The listing builds one solid part. Answer for the finished solid, in the listing's coordinates (mm). Coordinates: 2 decimals unless noted, no trailing zeros. Return JSON: item names as keys, results as strings.
Autodesk Inventor part; units mm, degrees
ref_plane "Work Plane1" through (0, 1.5, 0) normal (0, 1, 0) x (1, 0, 0)
ref_plane "YZ Plane" through (0, 0, 0) normal (1, 0, 0) x (0, 1, 0)
ref_plane "XZ Plane" through (0, 0, 0) normal (0, 1, 0) x (-1, 0, 0)
sketch "Sketch1" plane through (0, 0, 0) normal (0, 1, 0) x (-1, 0, 0)
  circle A0 centre (0, 0) radius 7.5
  dimension "d0" = 15
extrude "Extrusion1" add sketch "Sketch1" along normal blind 1
ref_plane "Work Plane1" through (0, 1.5, 0) normal (0, 1, 0) x (1, 0, 0)
sketch "Sketch3" plane through (0, 1.5, 0) normal (0, 1, 0) x (1, 0, 0)
  circle A0 centre (0, 0) radius 1.6
  dimension "d7" = 3.2
extrude "Extrusion3" cut sketch "Sketch3" against normal up to surface (1.5 mm away)
fillet "Fillet2" radius 0.5 2 edges at (7.5, 0, 0) (7.5, 1, 0)
chamfer "Chamfer2" distance 0.25 angle 45 2 edges at (-1.6, 0, 0) (-1.6, 1, 0)
properties part number "BoxWasher"
1. Consider line 1 (Z direction, x = 0, y = 0.55); line 2 (X direction, y = 0.15, z = 5.75); line 3 (Z direction, x = -3, y = 0.65). Determine where each line is inside the solid, lowest interval first. Write a range as from..to.
Answer block:
{"line 1": "z = -7.5..-1.6, 1.6..7.5", "line 2": "x = -4.59..4.59", "line 3": "z = -6.85..6.85"}
2. This flat-tipped pin is pushed along its axis until it touches: pin 1 Ø3.5 at (x, z) = (0, 0) entering from +Y. Where does it stop, or does it pass through?
Answer block:
{"pin 1": "stops at y = 0.9"}
3. Determine the mould class of faces 1 (the face through (-1.27, 0.5, 0.97)), 2 (the face through (-1.5, 1, -1.5)) for opening direction Z: pulls with the +Z half, pulls with the -Z half, needs draft (parallel to the pull), parting line crosses it, or undercut.
Answer block:
{"face 1": "undercut", "face 2": "needs draft"}
